```python
from build123d import *

# Parameters (mm, degrees)
SKETCH1_W           = 41.4
SKETCH1_H           = 41.4
SKETCH1_W_2         = 25.4
SKETCH1_H_2         = 25.4
BOSS_EXTRUDE1_DEPTH = 30
SKETCH2_W           = 41.4
SKETCH2_H           = 41.4
BOSS_EXTRUDE2_DEPTH = 10
BOSS_EXTRUDE3_DEPTH = 41.4
SKETCH4_R           = 2.5
CUT_EXTRUDE1_DEPTH  = 41.4
CUT_EXTRUDE2_REACH  = 78.334
SKETCH5_R           = 2.5
SKETCH6_R           = 4
CUT_EXTRUDE3_DEPTH  = 2
CUT_EXTRUDE4_START  = -2
SKETCH7_R           = 4
CUT_EXTRUDE4_DEPTH  = 2


with BuildPart() as part:
    # Sketch1 → Boss-Extrude1 (new body)
    with BuildSketch(Plane.XY):
        Rectangle(SKETCH1_W, SKETCH1_H)
        Rectangle(SKETCH1_W_2, SKETCH1_H_2, mode=Mode.SUBTRACT)
    extrude(amount=BOSS_EXTRUDE1_DEPTH)

    # Sketch2 → Boss-Extrude2 (add)
    with BuildSketch(Plane.XY.offset(30)):
        Rectangle(SKETCH2_W, SKETCH2_H)
    extrude(amount=BOSS_EXTRUDE2_DEPTH)

    # Sketch3 → Boss-Extrude3 (add)
    with BuildSketch(Plane(origin=(20.7, 0, 0), x_dir=(0, 0, -1), z_dir=(1, 0, 0))):
        with BuildLine():
            Line((-40, -20.7), (-40, 20.7))
            ThreePointArc((-40, 20.7), (-60.7, 0), (-40, -20.7))
        make_face()
    extrude(amount=-BOSS_EXTRUDE3_DEPTH)

    # Sketch4 → Cut-Extrude1 (cut)
    with BuildSketch(Plane(origin=(20.7, 0, 0), x_dir=(0, 0, -1), z_dir=(1, 0, 0))):
        with Locations((-40, 0)):
            Circle(SKETCH4_R)
    extrude(amount=-CUT_EXTRUDE1_DEPTH, mode=Mode.SUBTRACT)

    # Cut-Extrude2: up to this face of the body (flat: up to its plane)
    cut_extrude2_end = Plane(part.part.faces().sort_by_distance((20.7, 0, 28.219269494))[0])
    # Sketch5 → Cut-Extrude2 (cut, up to the picked face)
    with BuildSketch(Plane.ZY.offset(20.7), mode=Mode.PRIVATE) as cut_extrude2_sk1:
        with Locations((12.5, 0)):
            Circle(SKETCH5_R)
    cut_extrude2_tool1 = split(extrude(cut_extrude2_sk1.sketch, amount=-CUT_EXTRUDE2_REACH, mode=Mode.PRIVATE), bisect_by=cut_extrude2_end, keep=Keep.BOTH, mode=Mode.PRIVATE)
    add(cut_extrude2_tool1.solids().sort_by(Axis((-20.7, 0, 12.5), (1, 0, 0)))[0], mode=Mode.SUBTRACT)

    # Sketch6 → Cut-Extrude3 (cut)
    with BuildSketch(Plane.ZY.offset(20.7)):
        with Locations((12.5, 0)):
            Circle(SKETCH6_R)
    extrude(amount=-CUT_EXTRUDE3_DEPTH, mode=Mode.SUBTRACT)

    # Sketch7 → Cut-Extrude4 (cut)
    with BuildSketch(Plane(origin=(20.7, 0, 0), x_dir=(0, 0, -1), z_dir=(1, 0, 0)).offset(CUT_EXTRUDE4_START)):
        with Locations(Location((-12.5, 0, 0), (0, 0, 180))):
            Circle(SKETCH7_R)
    extrude(amount=CUT_EXTRUDE4_DEPTH, mode=Mode.SUBTRACT)


solid = part.part
```
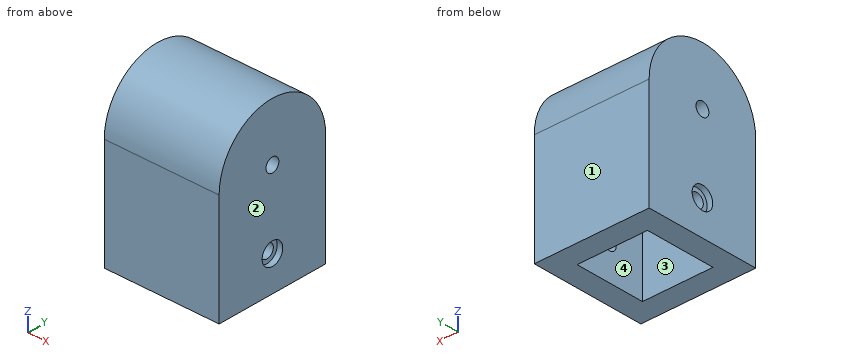
Can you work these out from the model? Positions are in its coordinate system, mm. Face numbers are marked on the shaded views. Round coordinates to 2 decimals unless told otherwise and drop trailing zeros. Loops run counter-clockwise (first coordinate to the right, second up) from the corner with the lowest first, then second, coordinate; pieces in that order, holes last. Notation, with made-up numbers: M -23.75,66.5 L 24.25,66.5 A18 ccw 24.25,100.5 Z; hole C 21.5,68 d11. An arc over 180 degrees is marked long. Write item = value, one per line. Start each with the question number.
(1) Suppose I cut it at C-C on x = -4. Write out the boundary of the cut face in (y, z).
(2) Suppose I cut it at A-A on y = 0. Write out the boundary of the cut face in (x, z).
(3) I'm going to push flat-ended pins straight in: P1, Ø6.5, axis at y = 1, z = 13, coming from the +X side; P2, Ø4.5, axis at y = 0, z = 40, coming from the -X side; P3, Ø1, axis at x = -14, y = 11, coming from the +Z side; P4, Ø4, axis at x = -13.5, y = -14, coming from the +Z side. Where does each tip first touch, or does it pass through?
(4) If we mould it in two halves opening along X, with no side actions, what happens to the marked faces 1, 2, 3 and 4? For each: released by +X, released by -X, zero draft, split by the parting line, or undercut.
(5) Suppose I cut it at B-B on z = 12.5. Write out the boundary of the cut face in (x, y).
(6) I need wall thicknesses on line 1 along Y through (x, z) = (0, 28); line 2 along Y through (x, z) = (10, 40). Which ranges of each line are inside material? Lowest first, please.
(7) Suppose I cut it at D-D on z = 5.5. Write out the boundary of the cut face in (x, y).
Answer block:
q1.outline = M -20.7,0 L -12.7,0 L -12.7,30 L 12.7,30 L 12.7,0 L 20.7,0 L 20.7,40 A20.7 ccw -20.7,40 Z; hole C 0,40 d5
q2.outline = M -20.7,0 L -12.7,0 L -12.7,10 L -18.7,10 L -18.7,8.5 L -20.7,8.5 Z; M -20.7,16.5 L -18.7,16.5 L -18.7,15 L -12.7,15 L -12.7,30 L 12.7,30 L 12.7,15 L 18.7,15 L 18.7,16.5 L 20.7,16.5 L 20.7,37.5 L -20.7,37.5 Z; M -20.7,42.5 L 20.7,42.5 L 20.7,60.7 L -20.7,60.7 Z; M 12.7,0 L 20.7,0 L 20.7,8.5 L 18.7,8.5 L 18.7,10 L 12.7,10 Z
q3.P1 = 20.7
q3.P2 = through
q3.P3 = 57.84
q3.P4 = 56.87
q4.face_1 = zero draft
q4.face_2 = released by +X
q4.face_3 = undercut
q4.face_4 = undercut
q5.outline = M -20.7,-20.7 L 20.7,-20.7 L 20.7,-4 L 18.7,-4 L 18.7,-2.5 L 12.7,-2.5 L 12.7,-12.7 L -12.7,-12.7 L -12.7,-2.5 L -18.7,-2.5 L -18.7,-4 L -20.7,-4 Z; M -20.7,4 L -18.7,4 L -18.7,2.5 L -12.7,2.5 L -12.7,12.7 L 12.7,12.7 L 12.7,2.5 L 18.7,2.5 L 18.7,4 L 20.7,4 L 20.7,20.7 L -20.7,20.7 Z
q6.line_1 = -20.7 to -12.7, 12.7 to 20.7
q6.line_2 = -20.7 to -2.5, 2.5 to 20.7
q7.outline = M -20.7,-20.7 L 20.7,-20.7 L 20.7,20.7 L -20.7,20.7 Z; hole M -12.7,-12.7 L 12.7,-12.7 L 12.7,12.7 L -12.7,12.7 Z
